from build123d import *

# Parameters (mm, degrees)
SKETCH1_W           = 9
SKETCH1_H           = 8
BOSS_EXTRUDE1_DEPTH = 3
SKETCH2_W           = 3
SKETCH2_H           = 5
BOSS_EXTRUDE2_DEPTH = 3
SKETCH3_R           = 1.016
CUT_EXTRUDE1_DEPTH  = 4


with BuildPart() as part:
    # Sketch1 → Boss-Extrude1 (new body)
    with BuildSketch(Plane(origin=(0, 0, 0), x_dir=(1, 0, 0), z_dir=(0, 1, 0))):
        Rectangle(SKETCH1_W, SKETCH1_H)
    extrude(amount=BOSS_EXTRUDE1_DEPTH)

    # Sketch2 → Boss-Extrude2 (add)
    with BuildSketch(Plane(origin=(0, 3, 0), x_dir=(1, 0, 0), z_dir=(0, 1, 0))):
        with Locations((-6, 0)):
            Rectangle(SKETCH2_W, SKETCH2_H)
    extrude(amount=-BOSS_EXTRUDE2_DEPTH)

    # Sketch3 → Cut-Extrude1 (cut, through all)
    with BuildSketch(Plane(origin=(0, 3, 0), x_dir=(1, 0, 0), z_dir=(0, 1, 0))):
        Circle(SKETCH3_R)
    extrude(amount=-CUT_EXTRUDE1_DEPTH, mode=Mode.SUBTRACT)


solid = part.part
CAD build for the part. Positions are in the model's coordinates, mm. A direction names the side the tool comes from. Round coordinates to 2 decimals unless told otherwise and drop trailing zeros. Loops run counter-clockwise (first coordinate to the right, second up) from the corner with the lowest first, then second, coordinate; pieces in that order, holes last. Notation, with made-up numbers: (81.5, 8.25) - (133.5, 8.25) arc R18 cw to (133.5, 18.25) - close; hole circle Ø4 at (48.25, 60.5). An arc over 180 degrees is marked (long way). Put each result on its own line as item: value.
1. Slice it at B-B on z = 0. List the corners of the cut face in (x, y), and give its area (3 significant figures).
Geometry check:
outline: (-7.5, 0) - (-1.02, 0) - (-1.02, 3) - (-7.5, 3) - close; (1.02, 0) - (4.5, 0) - (4.5, 3) - (1.02, 3) - close
area: 29.9 mm²
2. Slice it at C-C on x = 0. List the corners of the cut face in (y, z), and give its area (3 significant figures).
Geometry check:
outline: (0, -4) - (3, -4) - (3, -1.02) - (0, -1.02) - close; (0, 1.02) - (3, 1.02) - (3, 4) - (0, 4) - close
area: 17.9 mm²
3. 3-axis set-ups, long thin cutter, end or side, ignore diameter. For faces 1 (the flat face through (-4.5, 1, 3)), 2 (the flat face through (-6, 2, -2.5)), 3 (the flat face through (0, 1, 4)): which of +Z, -Z, +X, -X, +Y, -Y reach the whole face in a straight line?
Geometry check:
face 1: +Z, -X, +Y, -Y
face 2: -Z, -X, +Y, -Y
face 3: +Z, +X, -X, +Y, -Y
4. Two-plate mould, pull along Z, no slides. Class faces 4 (the flat face through (4.5, 1, 0)), 5 (the flat face through (-6, 2, 2.5)), 6 (the cylindrical face through (-0.22, 1.52, 0.99)): released by +Z, released by -Z, zero draft, split by the parting line, or undercut.
Geometry check:
face 4: zero draft
face 5: released by +Z
face 6: undercut
5. Wall check: line 1 (X direction, y = 2.25, z = 0); line 2 (Z direction, x = 0, y = 2.15); line 3 (X direction, y = 2.35, z = 3). Give the ranges that are in metal, low to high.
Geometry check:
line 1: -7.5 to -1.02, 1.02 to 4.5
line 2: -4 to -1.02, 1.02 to 4
line 3: -4.5 to 4.5
6. Pin check, flat tips, straight feed: P1, Ø1.2, axis at y = 1.5, z = 3.5, coming from the -X side; P2, Ø0.9, axis at x = -6, y = 1, coming from the +Z side; P3, Ø1.5, axis at x = -6, y = 2, coming from the -Z side; P4, Ø1.2, axis at x = 0, z = 0, coming from the -Y side. Stop position of each tip, or through.
Geometry check:
P1: x = -4.5
P2: z = 2.5
P3: z = -2.5
P4: through
7. Slice it at D-D on z = 3. List the corners of the cut face in (x, y), and give its area (3 significant figures).
Geometry check:
outline: (-4.5, 0) - (4.5, 0) - (4.5, 3) - (-4.5, 3) - close
area: 27.0 mm²
8. Slice it at A-A on y = 1.7. List the corners of the cut face in (x, z).
Geometry check:
outline: (-7.5, -2.5) - (-4.5, -2.5) - (-4.5, -4) - (4.5, -4) - (4.5, 4) - (-4.5, 4) - (-4.5, 2.5) - (-7.5, 2.5) - close; hole circle Ø2.03 at (0, 0)
